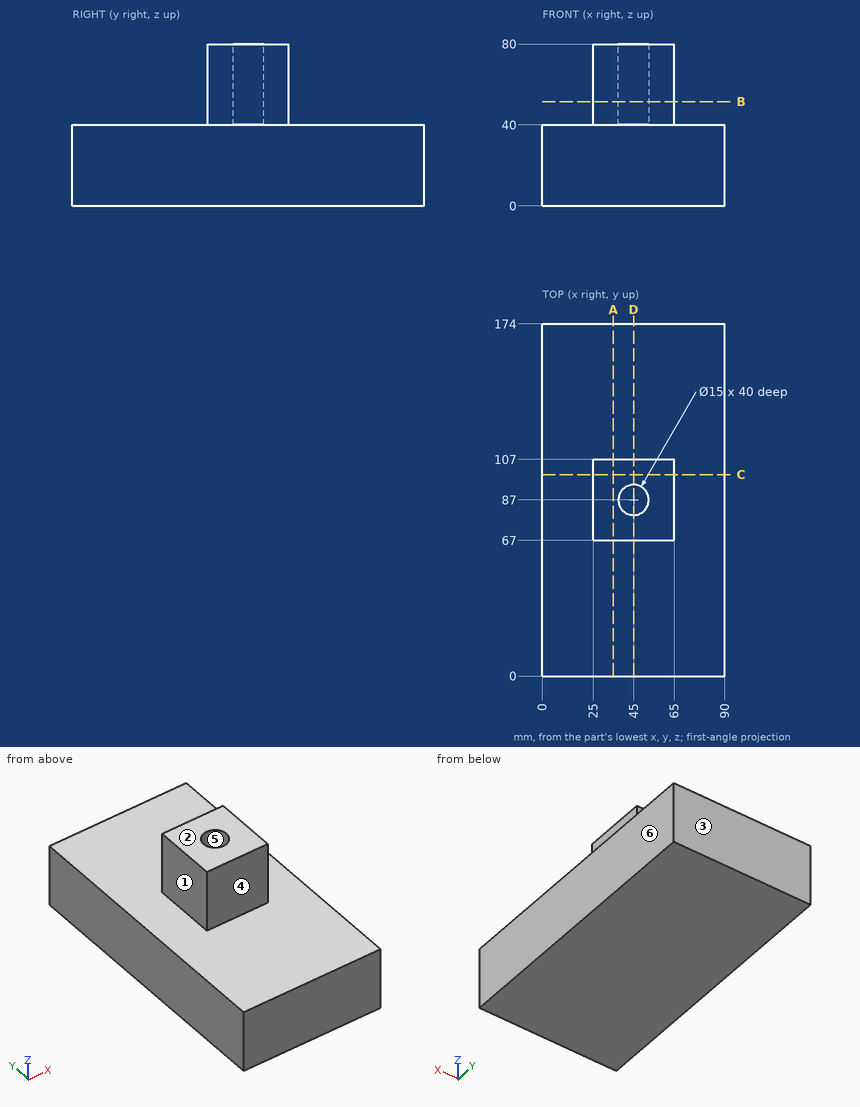
Job drawing, mm, ordinate dimensions from the low corner. One solid piece. A direction names the side the tool comes from. Give positions to 0.01 mm unless a question says otherwise; leave off trailing zeros. Order: outer loops, then holes, each group sorted by start corner. A loop starts at its lowest first (then second) coordinate and runs counter-clockwise, first axis right, second up. Notation, with made-up numbers: M 57,65 L 112,65 A16 cw 112,70 Z; hole C 16.25,13 d6. An arc over 180 degrees is marked long. Put each result on its own line as item: value. Start each with the question number.
(1) Band-saw the part on B-B on z = 51.5. Give the cut face in (x, y).
(2) Drill centre lines: L1, parallel to Y at x = 45, z = 50; L2, parallel to Z at x = 11, y = 70; L3, parallel to Y at x = 53, z = 42.5. Where is each one in solid material? Low to high. Write a range as [from, to].
(3) Band-saw the part on D-D on x = 45. Give the cut face in (y, z), then the cut area to 3 significant figures.
(4) Tool access for the marked faces 1 and 2: list every direction of +Z, -Z, +X, -X, +Y, -Y with a clear straight run to the whole face (end or side of a thin tool).
(5) Pin check, flat tips, straight feed: pin 1 Ø8 at (x, y) = (11, 32.5) entering from +Z; pin 2 Ø12 at (y, z) = (90.5, 64.5) entering from +X; pin 3 Ø20 at (y, z) = (91.5, 67.5) entering from -X. Stop position of each tip, or through.
(6) Band-saw the part on C-C on y = 99.5. Give the cut face in (x, z), then the cut area to 3 significant figures.
(7) Band-saw the part on A-A on x = 35. Give the cut face in (y, z), then the cut area to 3 significant figures.
(8) Pull direction Y, two halves, no side cores. Call the marked faces 3, 4, 5 and 6: released by +Y, released by -Y, zero draft, split by the parting line, or undercut.
Results below:
1. outline: M 25,67 L 65,67 L 65,107 L 25,107 Z; hole C 45,87 d15
2. L1: y = [67, 79.5], [94.5, 107]
2. L2: z = [0, 40]
2. L3: y = [67, 107]
3. outline: M 0,0 L 174,0 L 174,40 L 107,40 L 107,80 L 94.5,80 L 94.5,40 L 79.5,40 L 79.5,80 L 67,80 L 67,40 L 0,40 Z
3. area: 7,960 mm2
4. face 1: +Z, -X, +Y, -Y
4. face 2: +Z, +X, -X, +Y, -Y
5. pin 1: stops at z = 40
5. pin 2: stops at x = 65
5. pin 3: stops at x = 25
6. outline: M 0,0 L 90,0 L 90,40 L 65,40 L 65,80 L 25,80 L 25,40 L 0,40 Z
6. area: 5,200 mm2
7. outline: M 0,0 L 174,0 L 174,40 L 107,40 L 107,80 L 67,80 L 67,40 L 0,40 Z
7. area: 8,560 mm2
8. face 3: released by +Y
8. face 4: released by -Y
8. face 5: undercut
8. face 6: zero draft
